```python
from build123d import *

# Parameters (mm, degrees)
SKETCH_1_W          = 143
SKETCH_1_H          = 6
SKETCH_1_R          = 1.6
EXTRUDE_1_DEPTH     = 4
SKETCH_2_W          = 107
SKETCH_2_H          = 2
EXTRUDE_2_DEPTH     = 40
SKETCH_3_W          = 107
SKETCH_3_H          = 15
CUT_EXTRUDE_1_DEPTH = 145.696233538
FILLET_2_R          = 1


with BuildPart() as part:
    # 草图1 → 凸台-拉伸1 (new body)
    with BuildSketch(Plane(origin=(0, 0, 0), x_dir=(1, 0, 0), z_dir=(0, 1, 0))):
        with Locations((67.5, 0)):
            Rectangle(SKETCH_1_W, SKETCH_1_H)
        with Locations(Location((0, 0, 0), (0, 0, 270))):
            Circle(SKETCH_1_R, mode=Mode.SUBTRACT)
        with Locations(Location((10, 0, 0), (0, 0, 270))):
            Circle(SKETCH_1_R, mode=Mode.SUBTRACT)
        with Locations(Location((125, 0, 0), (0, 0, 270))):
            Circle(SKETCH_1_R, mode=Mode.SUBTRACT)
        with Locations(Location((135, 0, 0), (0, 0, 270))):
            Circle(SKETCH_1_R, mode=Mode.SUBTRACT)
    extrude(amount=EXTRUDE_1_DEPTH)

    # 草图2 → 凸台-拉伸2 (add)
    with BuildSketch(Plane.XZ):
        with Locations((67.5, -2)):
            Rectangle(SKETCH_2_W, SKETCH_2_H)
    extrude(amount=EXTRUDE_2_DEPTH)

    # 草图3 → 切除-拉伸1 (cut, through all)
    with BuildSketch(Plane.XY.offset(-1)):
        with Locations((67.5, -32.5)):
            Rectangle(SKETCH_3_W, SKETCH_3_H)
    extrude(amount=-CUT_EXTRUDE_1_DEPTH, mode=Mode.SUBTRACT)

    # 圆角2
    fillet_2_edges = [part.edges().sort_by_distance(p)[0] for p in [
        (14, 0, -2),
        (121, 0, -2),
        (14, -25, -2),
        (121, -25, -2),
        (-4, 2, -3),
        (139, 2, -3),
        (139, 2, 3),
        (-4, 2, 3),
    ]]
    fillet(fillet_2_edges, radius=FILLET_2_R)


solid = part.part
```
The listing builds one solid part. Answer for the finished solid, in the listing's coordinates (mm). A direction names the side the tool comes from. Round coordinates to 2 decimals unless told otherwise and drop trailing zeros. Loops run counter-clockwise (first coordinate to the right, second up) from the corner with the lowest first, then second, coordinate; pieces in that order, holes last. Notation, with made-up numbers: (-23.75, 64) - (-9.75, 64) arc R18 cw to (-9.75, 93) - close; hole circle Ø4 at (62, -29). An arc over 180 degrees is marked (long way). Use one line per item in the form item = value. Start each with the question number.
1. Given pin 1 Ø4 at (x, y) = (12.5, -19) entering from +Z; pin 2 Ø2 at (y, z) = (-14, -1.5) entering from -X; pin 3 Ø0.6 at (y, z) = (-16.5, -2) entering from +X, each flat-ended and moving along its own axis, determine where each tip first touches the part or whether it passes through.
2. A tool of negligible diameter and unlimited length cuts with its end or side. For faces 4 (the face through (67, -12, -1)), 5 (the face through (-4, 2, 0)), from which of +Z, -Z, +X, -X, +Y, -Y can it reach the whole face along a straight path? Write none if from no direction.
3. For a pull along Z with two mould halves and no side action, classify faces 1 (the face through (-0.97, 1.97, -1.27)), 2 (the face through (67, 2, 3)), 3 (the face through (139, 2, 0)) as pulls with the +Z half, pulls with the -Z half, needs draft (parallel to the pull), parting line crosses it, or undercut.
4. The part is cut by section C-C on x = 92.5. Determine the outline of the cut face in (y, z).
5. Consider line 1 (X direction, y = 2.8, z = 0); line 2 (X direction, y = 0.25, z = -0.45); line 3 (Z direction, x = 135, y = 1.2). Determine where each line is inside the solid, lowest interval first. Write a range as [from, to].
6. The part is cut by section D-D on y = -5. Determine the outline of the cut face in (x, z).
7. The part is cut by section A-A on x = 0. Determine the outline of the cut face in (y, z).
8. The part is cut by section B-B on z = 0. Determine the outline of the cut face in (x, y), then the cut area to 3 significant figures.
Geometry check:
q1.pin_1 = -1
q1.pin_2 = 14
q1.pin_3 = 121
q2.face_4 = +Z, +X, -X, -Y
q2.face_5 = +Z, -Z, -X, +Y, -Y
q3.face_1 = undercut
q3.face_2 = pulls with the +Z half
q3.face_3 = needs draft
q4.outline = (-25, -3) - (4, -3) - (4, 3) - (0, 3) - (0, -1) - (-25, -1) - close
q5.line_1 = [-4, -1.6], [1.6, 8.4], [11.6, 123.4], [126.6, 133.4], [136.6, 139]
q5.line_2 = [-4, -1.54], [1.54, 8.46], [11.54, 123.46], [126.54, 133.46], [136.54, 139]
q5.line_3 = [-3, -1.6], [1.6, 3]
q6.outline = (14, -3) - (121, -3) - (121, -1) - (14, -1) - close
q7.outline = (0, -3) - (4, -3) - (4, -1.6) - (0, -1.6) - close; (0, 1.6) - (4, 1.6) - (4, 3) - (0, 3) - close
q8.outline = (-4, 0) - (-1.6, 0) - (-1.6, 4) - (-4, 4) - close; (1.6, 0) - (8.4, 0) - (8.4, 4) - (1.6, 4) - close; (11.6, 0) - (123.4, 0) - (123.4, 4) - (11.6, 4) - close; (126.6, 0) - (133.4, 0) - (133.4, 4) - (126.6, 4) - close; (136.6, 0) - (139, 0) - (139, 4) - (136.6, 4) - close
q8.area = 521 mm^2
